Part model, mm, in its own coordinate system. Face numbers are marked on the shaded views. A direction names the side the tool comes from. Round coordinates to 2 decimals unless told otherwise and drop trailing zeros. Loops run counter-clockwise (first coordinate to the right, second up) from the corner with the lowest first, then second, coordinate; pieces in that order, holes last. Notation, with made-up numbers: (-24, -7) -> (-7, -7) arc R15 ccw to (-7, 22) -> close; hole circle Ø9 at (79.25, 36). An arc over 180 degrees is marked (long way). Answer as CSV lines item,"result".
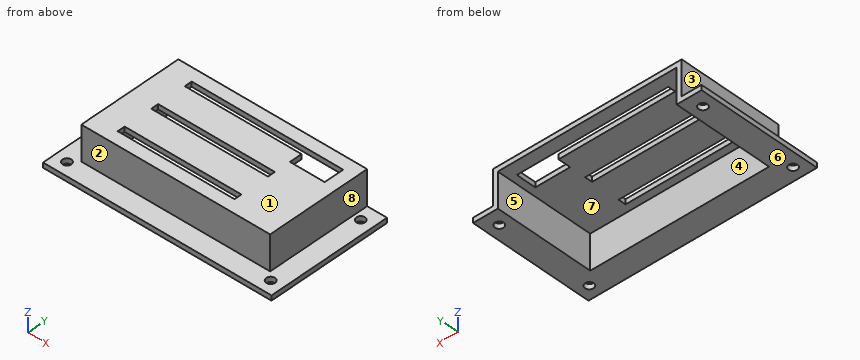
from build123d import *

# Parameters (mm, degrees)
SKETCH031_R   = 1.75
PAD017_DEPTH  = 2
PAD018_DEPTH  = 12
SKETCH033_W   = 76
SKETCH033_H   = 42
SKETCH033_W_2 = 47
SKETCH033_H_2 = 3
PAD019_DEPTH  = 2


with BuildPart() as part:
    # Sketch031 → Pad017 (new body)
    with BuildSketch(Plane.XY):
        Polygon((10, 0), (0, 0), (0, -50), (92, -50), (92, 0), (82, 0), (82, -40), (10, -40), align=None)
        with Locations((5, -45)):
            Circle(SKETCH031_R, mode=Mode.SUBTRACT)
        with Locations((87, -45)):
            Circle(SKETCH031_R, mode=Mode.SUBTRACT)
        with Locations((87, -6)):
            Circle(SKETCH031_R, mode=Mode.SUBTRACT)
        with Locations((5, -6)):
            Circle(SKETCH031_R, mode=Mode.SUBTRACT)
    extrude(amount=PAD017_DEPTH)

    # Sketch032 (on Face14 of Pad017) → Pad018 (join)
    with BuildSketch(Plane.XY.offset(2)):
        Polygon((10, 0), (10, -40), (82, -40), (82, 0), (84, 0), (84, -42), (8, -42), (8, 0), align=None)
    extrude(amount=PAD018_DEPTH)

    # Sketch033 (on Face18 of Pad018) → Pad019 (join)
    with BuildSketch(Plane.XY.offset(14)):
        with Locations((46, -21)):
            Rectangle(SKETCH033_W, SKETCH033_H)
        Polygon((18, -5), (74, -5), (79, -5), (79, -13), (65, -13), (65, -8), (18, -8), align=None, mode=Mode.SUBTRACT)
        with Locations((41.5, -21)):
            Rectangle(SKETCH033_W_2, SKETCH033_H_2, mode=Mode.SUBTRACT)
        with Locations((41.5, -35.5)):
            Rectangle(SKETCH033_W_2, SKETCH033_H_2, mode=Mode.SUBTRACT)
    extrude(amount=PAD019_DEPTH)


with BuildPart() as part_1:
    # Body015 placement: moved
    add(part.part.moved(Location((0, 125, 0))))


solid = part_1.part
Q1. Two-plate mould, pull along X, no slides. Class the marked faces 5, 6, 7 and 8: pulls with the +X half, pulls with the -X half, needs draft (parallel to the pull), parting line crosses it, or undercut.
Geometry results:
face 5,"undercut"
face 6,"needs draft"
face 7,"undercut"
face 8,"pulls with the +X half"
Q2. Saw through at B-B, the plane x = 27.5. Write the cut outline in (y, z), then the cut area to 3 significant figures.
Geometry results:
outline,"(75, 0) -> (85, 0) -> (85, 14) -> (88, 14) -> (88, 16) -> (83, 16) -> (83, 2) -> (75, 2) -> close; (91, 14) -> (102.5, 14) -> (102.5, 16) -> (91, 16) -> close; (105.5, 14) -> (117, 14) -> (117, 16) -> (105.5, 16) -> close; (120, 14) -> (125, 14) -> (125, 16) -> (120, 16) -> close"
area,"110 mm2"
Q3. Saw through at C-C, the plane z = 5.5. Write the cut outline in (x, y).
Geometry results:
outline,"(8, 83) -> (84, 83) -> (84, 125) -> (82, 125) -> (82, 85) -> (10, 85) -> (10, 125) -> (8, 125) -> close"
Q4. Drop flat-ended pins along their axis: P1, Ø2, axis at y = 119, z = 15, coming from the +X side; P2, Ø1, axis at y = 104, z = 15.5, coming from the -X side; P3, Ø1, axis at x = 38.5, z = 14.5, coming from the -Y side. Give the stop position or say it passes through.
Geometry results:
P1,"x = 84"
P2,"x = 8"
P3,"y = 83"
Q5. Drill centre lines: line 1 along Y through (x, z) = (87, 1.4); line 2 along X through (y, z) = (80, 0.6); line 3 along X through (y, z) = (107.5, 12.5). Where is each one in solid material? Low to high.
Geometry results:
line 1,"75 to 78.25, 81.75 to 117.25, 120.75 to 125"
line 2,"0 to 3.25, 6.75 to 85.25, 88.75 to 92"
line 3,"8 to 10, 82 to 84"
Q6. Saw through at D-D, the plane x = 5. Write the cut outline in (y, z).
Geometry results:
outline,"(75, 0) -> (78.25, 0) -> (78.25, 2) -> (75, 2) -> close; (81.75, 0) -> (117.25, 0) -> (117.25, 2) -> (81.75, 2) -> close; (120.75, 0) -> (125, 0) -> (125, 2) -> (120.75, 2) -> close"
Q7. Which spindle directions (+Z, -Z, +X, -X, +Y, -Y) get a long thin tool onto all of the face, cutting with end or side? Do the marked faces 1, 2, 3 and 4. Say none if no direction does.
Geometry results:
face 1,"+Z, +X, -X, +Y, -Y"
face 2,"+Z, +X, -X, -Y"
face 3,"+Z, -X, +Y, -Y"
face 4,"-Z, +Y"
Q8. Saw through at A-A, the plane y = 80. Write the cut outline in (x, z), then the cut area to 3 significant figures.
Geometry results:
outline,"(0, 0) -> (3.25, 0) -> (3.25, 2) -> (0, 2) -> close; (6.75, 0) -> (85.25, 0) -> (85.25, 2) -> (6.75, 2) -> close; (88.75, 0) -> (92, 0) -> (92, 2) -> (88.75, 2) -> close"
area,"170 mm2"
